from build123d import *

# Parameters (mm, degrees)
SKETCH1_R           = 1.35
SKETCH1_R_2         = 12.095
SKETCH1_W           = 11
SKETCH1_H           = 69
BOSS_EXTRUDE2_DEPTH = 3.175
FILLET1_R           = 2


with BuildPart() as part:
    # Sketch1 → Boss-Extrude2 (new body)
    with BuildSketch(Plane(origin=(0, 0, 0), x_dir=(1, 0, 0), z_dir=(0, 1, 0))):
        with BuildLine():
            ThreePointArc((32.995567884, -67.352004425), (0, 75), (-32.995567884, -67.352004425))
            ThreePointArc((-32.995567884, -67.352004425), (0, -48.302004425), (32.995567884, -67.352004425))
        make_face()
        with Locations((-42.910067426, 11.1)):
            Circle(SKETCH1_R, mode=Mode.SUBTRACT)
        with Locations((-42.910067426, -11.1)):
            Circle(SKETCH1_R, mode=Mode.SUBTRACT)
        with Locations((-11.160067426, -11.1)):
            Circle(SKETCH1_R, mode=Mode.SUBTRACT)
        with Locations((-11.160067426, 11.1)):
            Circle(SKETCH1_R, mode=Mode.SUBTRACT)
        with Locations((11.160067426, 11.1)):
            Circle(SKETCH1_R, mode=Mode.SUBTRACT)
        with Locations((11.160067426, -11.1)):
            Circle(SKETCH1_R, mode=Mode.SUBTRACT)
        with Locations((42.910067426, -11.1)):
            Circle(SKETCH1_R, mode=Mode.SUBTRACT)
        with Locations((42.910067426, 11.1)):
            Circle(SKETCH1_R, mode=Mode.SUBTRACT)
        with Locations((26.905821676, -20.904643604)):
            Circle(SKETCH1_R_2, mode=Mode.SUBTRACT)
        with Locations((19, 49)):
            Circle(SKETCH1_R_2, mode=Mode.SUBTRACT)
        with Locations((0, 29.793589551)):
            Circle(SKETCH1_R_2, mode=Mode.SUBTRACT)
        with Locations((0, -25.409190322)):
            Circle(SKETCH1_R_2, mode=Mode.SUBTRACT)
        with Locations((29.939937248, 24.651901309)):
            Circle(SKETCH1_R_2, mode=Mode.SUBTRACT)
        with Locations((-26.905821676, -20.904643604)):
            Circle(SKETCH1_R_2, mode=Mode.SUBTRACT)
        with Locations((-29.939937248, 24.651901309)):
            Circle(SKETCH1_R_2, mode=Mode.SUBTRACT)
        with Locations((-33.21799214, 49)):
            Circle(SKETCH1_R, mode=Mode.SUBTRACT)
        with Locations((-4.78200786, 49)):
            Circle(SKETCH1_R, mode=Mode.SUBTRACT)
        with Locations((4.78200786, 49)):
            Circle(SKETCH1_R, mode=Mode.SUBTRACT)
        with Locations((-42.910067426, 18.234848025)):
            Circle(SKETCH1_R, mode=Mode.SUBTRACT)
        with Locations((42.910067426, 18.234848025)):
            Circle(SKETCH1_R, mode=Mode.SUBTRACT)
        with Locations((-19, 49)):
            Circle(SKETCH1_R_2, mode=Mode.SUBTRACT)
        with Locations((45.13872464, 31.997163897)):
            Circle(SKETCH1_R, mode=Mode.SUBTRACT)
        with Locations((-45.13872464, 31.997163897)):
            Circle(SKETCH1_R, mode=Mode.SUBTRACT)
        with Locations((13.346873881, 34.693819966)):
            Circle(SKETCH1_R, mode=Mode.SUBTRACT)
        with Locations((-6.55476095, -38.026099982)):
            Circle(SKETCH1_R, mode=Mode.SUBTRACT)
        with Locations((-13.346873881, 34.693819966)):
            Circle(SKETCH1_R, mode=Mode.SUBTRACT)
        with Locations((10.597026674, -15.930038136)):
            Circle(SKETCH1_R, mode=Mode.SUBTRACT)
        with Locations((-38.234289702, -39.23697625)):
            Circle(SKETCH1_R, mode=Mode.SUBTRACT)
        with Locations((-43.684644625, -41.077803557)):
            Circle(SKETCH1_R, mode=Mode.SUBTRACT)
        with Locations((-43.684644625, 41.077803557)):
            Circle(SKETCH1_R, mode=Mode.SUBTRACT)
        with Locations((43.684644625, -41.077803557)):
            Circle(SKETCH1_R, mode=Mode.SUBTRACT)
        with Locations((33.21799214, 49)):
            Circle(SKETCH1_R, mode=Mode.SUBTRACT)
        with Locations((43.684644625, 41.077803557)):
            Circle(SKETCH1_R, mode=Mode.SUBTRACT)
        with Locations((-44.385223141, -22.074211772)):
            Circle(SKETCH1_R, mode=Mode.SUBTRACT)
        with Locations((41.601681906, -17.457756634)):
            Circle(SKETCH1_R, mode=Mode.SUBTRACT)
        with Locations((38.234289702, -39.23697625)):
            Circle(SKETCH1_R, mode=Mode.SUBTRACT)
        with Locations((58.910067426, 0.102907352)):
            Rectangle(SKETCH1_W, SKETCH1_H, mode=Mode.SUBTRACT)
        with Locations((-58.910067426, 0.102907352)):
            Rectangle(SKETCH1_W, SKETCH1_H, mode=Mode.SUBTRACT)
        with BuildLine():
            ThreePointArc((-5.853899988, 64.744946271), (0.003726822, 68.153564176), (5.857575472, 64.738461857))
            ThreePointArc((5.857575472, 64.738461857), (10.16, 61.422565207), (5.857575472, 58.106668557))
            ThreePointArc((5.857575472, 58.106668557), (0.003726822, 54.691566239), (-5.853899988, 58.100184144))
            ThreePointArc((-5.853899988, 58.100184144), (-10.167207264, 61.422565207), (-5.853899988, 64.744946271))
        make_face(mode=Mode.SUBTRACT)
    extrude(amount=BOSS_EXTRUDE2_DEPTH)

    # Fillet1
    fillet1_edges = [part.edges().sort_by_distance(p)[0] for p in [
        (-32.995567884, 1.5875, 67.352004425),
        (32.995567884, 1.5875, 67.352004425),
    ]]
    fillet(fillet1_edges, radius=FILLET1_R)


solid = part.part
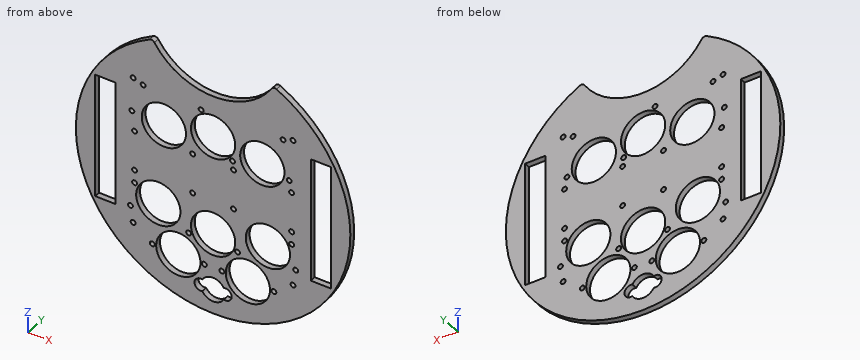
Read the model definition and answer for the solid it produces. Units are mm, in the model's axes. Round coordinates to 2 decimals unless told otherwise and drop trailing zeros. Write each loop counter-clockwise with the first axis right and the second up, starting at its lowest first coordinate (ties: lowest second). Pieces come first, ordered by that corner, then holes.
1. The part is cut by section D-D, the plane y = 1.25. State how many separate pieces and enclosed holes the cut face has, then the cut area to 3 significant figures.
2. Straight lines are drawn through the part: L1, parallel to X at y = 2.8, z = 39; L2, parallel to Z at x = 2.5, y = 1; L3, parallel to Z at x = -60, y = 0.5. For each, find the intervals that lie inside material, in ascending order.
3. The part is cut by section A-A, the plane z = 0. Determine the outline of the cut face in (x, y) (3 decimals).
4. Given pin 1 Ø1.5 at (x, y) = (-2.5, 2.5) entering from +Z; pin 2 Ø2 at (x, z) = (-6.55, 38.03) entering from +Y, each flat-ended and moving along its own axis, determine where each tip first touches the part or whether it passes through.
5. The part is cut by section C-C, the plane z = -27. Determine the outline of the cut face in (x, y) (3 decimals), then the cut area to 3 significant figures.
6. The part is cut by section B-B, the plane x = 0. Determine the outline of the cut face in (y, z) (3 decimals), then the cut area to 3 significant figures.
Values:
1. separate pieces: 1
1. enclosed holes: 39
1. area: 10,900 mm2
2. L1: x = -64.06 to -39.56, -36.91 to -7.49, -5.62 to 36.91, 39.56 to 64.06
2. L2: z = -74.96 to -67.67, -55.17 to -41.63, -17.96 to 13.58, 37.24 to 48.38
2. L3: z = -45 to -34.6, 34.4 to 45
3. outline: (-75, 0) - (-64.41, 0) - (-64.41, 3.175) - (-75, 3.175) - close; (-53.41, 0) - (53.41, 0) - (53.41, 3.175) - (-53.41, 3.175) - close; (64.41, 0) - (75, 0) - (75, 3.175) - (64.41, 3.175) - close
4. pin 1: stops at z = 48.44
4. pin 2: passes through
5. outline: (-69.971, 0) - (-64.41, 0) - (-64.41, 3.175) - (-69.971, 3.175) - close; (-53.41, 0) - (-41.805, 0) - (-41.805, 3.175) - (-53.41, 3.175) - close; (-18.075, 0) - (-11.768, 0) - (-11.768, 3.175) - (-18.075, 3.175) - close; (11.768, 0) - (18.075, 0) - (18.075, 3.175) - (11.768, 3.175) - close; (41.805, 0) - (53.41, 0) - (53.41, 3.175) - (41.805, 3.175) - close; (64.41, 0) - (69.971, 0) - (69.971, 3.175) - (64.41, 3.175) - close
5. area: 149 mm2
6. outline: (0, -75) - (3.175, -75) - (3.175, -68.154) - (0, -68.154) - close; (0, -54.692) - (3.175, -54.692) - (3.175, -41.889) - (0, -41.889) - close; (0, -17.699) - (3.175, -17.699) - (3.175, 13.314) - (0, 13.314) - close; (0, 37.504) - (3.175, 37.504) - (3.175, 48.302) - (0, 48.302) - close
6. area: 195 mm2
